Verification items for the finished model (mm, model axes). Face numbers are marked on the shaded views. Give positions to 0.01 mm unless a question says otherwise; leave off trailing zeros. Loops run counter-clockwise (first coordinate to the right, second up) from the corner with the lowest first, then second, coordinate; pieces in that order, holes last. Notation, with made-up numbers: (-34, 23) - (-20, 23) arc R34 ccw to (-20, 57) - close; hole circle Ø2 at (40.25, 30.5). An arc over 180 degrees is marked (long way). One line per question, with ' | ' between items. Start each with the question number.
1. Depth check by flat-ended pin: pin 1 Ø7.5 at (x, y) = (74, -12) entering from +Z; pin 2 Ø1.4 at (x, y) = (42.5, 33) entering from -Z; pin 3 Ø0.8 at (x, z) = (52, 2) entering from -Y. Enter the tip coordinate at first touch or a pass-through.
2. Section check C-C, the plane y = -29. Enter the section's corners in (x, z), then the cut area to 3 significant figures.
3. Section check D-D, the plane x = 9. Enter the section's corners in (y, z).
4. Section check A-A, the plane y = -2. Enter the section's corners in (x, z).
5. Mould release check, pull along Y, two halves, no side actions. Record for the marked faces 1 and 2: +Y half, -Y half, draft (parallel to the pull), parting line (faces both ways), or undercut.
6. Thickness scan on line 1 along Y through (x, z) = (40, 1.75); line 2 along Y through (x, z) = (58, 6.75); line 3 along X through (y, z) = (-29, 2.75). Record the ranges inside material, lowest first. Write a range as from..to.
7. Section check B-B, the plane x = 17. Enter the section's corners in (y, z).
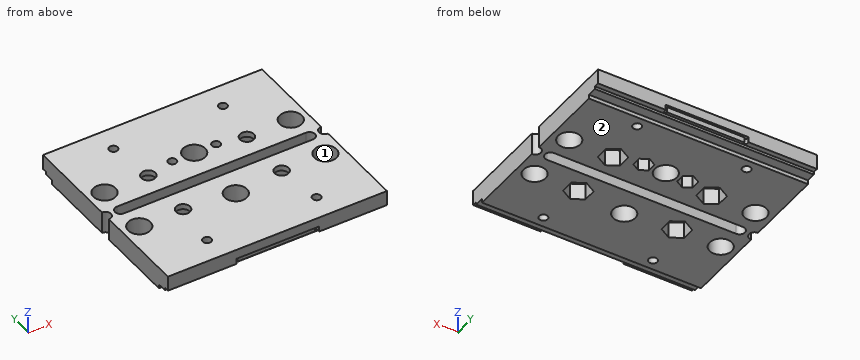
from build123d import *

# Parameters (mm, degrees)
SKETCH_2_W           = 80
SKETCH_2_H           = 34
SKETCH_2_R           = 4.05
EXTRUDE_1_DEPTH      = 8
SKETCH_3_R           = 2.55
CUT_EXTRUDE_1_DEPTH  = 88.292611371
CUT_EXTRUDE_2_DEPTH  = 88.292611371
SKETCH_5_R           = 1.55
CUT_EXTRUDE_3_DEPTH  = 88.292611371
CUT_EXTRUDE_4_DEPTH  = 6
CUT_EXTRUDE_5_DEPTH  = 4.5
SKETCH_25_R          = 1.55
CUT_EXTRUDE_13_DEPTH = 88.292611371
CUT_EXTRUDE_11_DEPTH = 2
EXTRUDE_2_DEPTH      = 8


with BuildPart() as part:
    # 草图2 → 凸台-拉伸1 (new body)
    with BuildSketch(Plane.XY):
        with Locations((40, 17)):
            Rectangle(SKETCH_2_W, SKETCH_2_H)
        with Locations((6, 8)):
            Circle(SKETCH_2_R, mode=Mode.SUBTRACT)
        with Locations((40, 10)):
            Circle(SKETCH_2_R, mode=Mode.SUBTRACT)
        with Locations((74, 8)):
            Circle(SKETCH_2_R, mode=Mode.SUBTRACT)
    extrude_1 = extrude(amount=EXTRUDE_1_DEPTH)

    # 草图3 → 切除-拉伸1 (cut, through all)
    with BuildSketch(Plane.XY.offset(8)):
        with Locations((22, 8)):
            Circle(SKETCH_3_R)
        with Locations((58, 8)):
            Circle(SKETCH_3_R)
    cut_extrude_1 = extrude(amount=-CUT_EXTRUDE_1_DEPTH, mode=Mode.SUBTRACT)

    # 草图4 → 切除-拉伸2 (cut, through all)
    with BuildSketch(Plane(origin=(80, 0, 0), x_dir=(0, 0, -1), z_dir=(1, 0, 0))):
        Polygon((-1.5, 32.2), (-2.5, 32.2), (-2.5, 34), (0, 34), (0, 28.8), (-1.5, 28.8), align=None)
    cut_extrude_2 = extrude(amount=-CUT_EXTRUDE_2_DEPTH, mode=Mode.SUBTRACT)

    # 草图5 → 切除-拉伸3 (cut, through all)
    with BuildSketch(Plane.XY.offset(8)):
        with Locations((48, 10)):
            Circle(SKETCH_5_R)
        with Locations((32, 10)):
            Circle(SKETCH_5_R)
    extrude(amount=-CUT_EXTRUDE_3_DEPTH, mode=Mode.SUBTRACT)

    # 草图7 → 切除-拉伸4 (cut)
    with BuildSketch(Plane(origin=(0, 0, 0), x_dir=(-1, 0, 0), z_dir=(0, 0, -1))):
        Polygon((-53.9, 5.632863896), (-53.9, 10.367136104), (-58, 12.734272207), (-62.1, 10.367136104), (-62.1, 5.632863896), (-58, 3.265727793), align=None)
        Polygon((-26.1, 5.632863896), (-22, 3.265727793), (-17.9, 5.632863896), (-17.9, 10.367136104), (-22, 12.734272207), (-26.1, 10.367136104), align=None)
    cut_extrude_4 = extrude(amount=-CUT_EXTRUDE_4_DEPTH, mode=Mode.SUBTRACT)

    # 草图8 → 切除-拉伸5 (cut)
    with BuildSketch(Plane(origin=(0, 0, 0), x_dir=(-1, 0, 0), z_dir=(0, 0, -1))):
        Polygon((-48, 6.709103466), (-45.15, 8.354551733), (-45.15, 11.645448267), (-48, 13.290896534), (-50.85, 11.645448267), (-50.85, 8.354551733), align=None)
        Polygon((-32, 6.709103466), (-29.15, 8.354551733), (-29.15, 11.645448267), (-32, 13.290896534), (-34.85, 11.645448267), (-34.85, 8.354551733), align=None)
    extrude(amount=-CUT_EXTRUDE_5_DEPTH, mode=Mode.SUBTRACT)

    # 草图25 → 切除-拉伸13 (cut, through all)
    with BuildSketch(Plane(origin=(0, 0, 0), x_dir=(-1, 0, 0), z_dir=(0, 0, -1))):
        with Locations((-60, 25)):
            Circle(SKETCH_25_R)
        with Locations((-20, 25)):
            Circle(SKETCH_25_R)
    cut_extrude_13 = extrude(amount=-CUT_EXTRUDE_13_DEPTH, mode=Mode.SUBTRACT)

    # 草图19 → 切除-拉伸11 (cut)
    with BuildSketch(Plane(origin=(0, 0, 2.5), x_dir=(-1, 0, 0), z_dir=(0, 0, -1))):
        with BuildLine():
            Line((-25, 34), (-55.247938178, 34))
            Line((-55.247938178, 34), (-55.247938178, 33.2))
            ThreePointArc((-55.247938178, 33.2), (-54.747938178, 32.7), (-54.247938178, 33.2))
            Line((-54.247938178, 33.2), (-26, 33.2))
            ThreePointArc((-26, 33.2), (-25.5, 32.7), (-25, 33.2))
            Line((-25, 33.2), (-25, 34))
        make_face()
    cut_extrude_11 = extrude(amount=-CUT_EXTRUDE_11_DEPTH, mode=Mode.SUBTRACT)

    # 草图22 → 凸台-拉伸2 (add)
    with BuildSketch(Plane.XY.offset(8)):
        with BuildLine():
            Line((0, -4), (5.5, -4))
            ThreePointArc((5.5, -4), (3.5, -2), (5.5, 0))
            Line((5.5, 0), (0, 0))
            ThreePointArc((0, 0), (2, -2), (0, -4))
        make_face()
        with BuildLine():
            Line((80, 0), (74.5, 0))
            ThreePointArc((74.5, 0), (76.5, -2), (74.5, -4))
            Line((74.5, -4), (80, -4))
            ThreePointArc((80, -4), (78, -2), (80, 0))
        make_face()
    extrude(amount=-EXTRUDE_2_DEPTH)

    # 镜向2: 凸台-拉伸1, 切除-拉伸1, 切除-拉伸2, 切除-拉伸4, 切除-拉伸13, 切除-拉伸11 across plane
    add(extrude_1.mirror(Plane(origin=(0, -2, 0), x_dir=(0, 0, 1), z_dir=(0, -1, 0))))
    add(cut_extrude_1.mirror(Plane(origin=(0, -2, 0), x_dir=(0, 0, 1), z_dir=(0, -1, 0))), mode=Mode.SUBTRACT)
    add(cut_extrude_2.mirror(Plane(origin=(0, -2, 0), x_dir=(0, 0, 1), z_dir=(0, -1, 0))), mode=Mode.SUBTRACT)
    add(cut_extrude_4.mirror(Plane(origin=(0, -2, 0), x_dir=(0, 0, 1), z_dir=(0, -1, 0))), mode=Mode.SUBTRACT)
    add(cut_extrude_13.mirror(Plane(origin=(0, -2, 0), x_dir=(0, 0, 1), z_dir=(0, -1, 0))), mode=Mode.SUBTRACT)
    add(cut_extrude_11.mirror(Plane(origin=(0, -2, 0), x_dir=(0, 0, 1), z_dir=(0, -1, 0))), mode=Mode.SUBTRACT)


solid = part.part
Results list:
1) pin 1: through | pin 2: z = 2.5 | pin 3: y = -36.2
2) outline: (0, 0) - (18.45, 0) - (18.45, 8) - (0, 8) - close; (21.55, 0) - (58.45, 0) - (58.45, 8) - (21.55, 8) - close; (61.55, 0) - (80, 0) - (80, 8) - (61.55, 8) - close | area: 590 mm²
3) outline: (-38, 2.5) - (-36.2, 2.5) - (-36.2, 1.5) - (-32.8, 1.5) - (-32.8, 0) - (-14.72, 0) - (-14.72, 8) - (-38, 8) - close; (-9.28, 0) - (-4, 0) - (-4, 8) - (-9.28, 8) - close; (0, 0) - (5.28, 0) - (5.28, 8) - (0, 8) - close; (10.72, 0) - (28.8, 0) - (28.8, 1.5) - (32.2, 1.5) - (32.2, 2.5) - (34, 2.5) - (34, 8) - (10.72, 8) - close
4) outline: (2, 0) - (3.5, 0) - (3.5, 8) - (2, 8) - close; (76.5, 0) - (78, 0) - (78, 8) - (76.5, 8) - close
5) face 1: undercut | face 2: draft
6) line 1: -36.2..-18.05, -9.95..-4, 0..5.95, 14.05..32.2 | line 2: -38..-14.55, -9.45..-4, 0..5.45, 10.55..34 | line 3: 0..18.45, 21.55..58.45, 61.55..80
7) outline: (-38, 2.5) - (-36.2, 2.5) - (-36.2, 1.5) - (-32.8, 1.5) - (-32.8, 0) - (-4, 0) - (-4, 8) - (-38, 8) - close; (0, 0) - (28.8, 0) - (28.8, 1.5) - (32.2, 1.5) - (32.2, 2.5) - (34, 2.5) - (34, 8) - (0, 8) - close
